```python
from build123d import *

# Parameters (mm, degrees)
SKETCH1_W                      = 912
SKETCH1_H                      = 225
BASE_FLANGE1_DEPTH             = 1.5
EDGE_FLANGE1_STRIP_W           = 10
EDGE_FLANGE1_STRIP_H           = 1.5
EDGE_FLANGE1_STRIP_CUT_DEPTH   = 912
EDGE_FLANGE1_STRIP_2_W         = 10
EDGE_FLANGE1_STRIP_2_H         = 1.5
EDGE_FLANGE1_STRIP_CUT_2_DEPTH = 912
EDGE_FLANGE1_DEPTH             = 912
EDGE_FLANGE1_BEND_DEPTH        = 912
EDGE_FLANGE2_STRIP_W           = 10
EDGE_FLANGE2_STRIP_H           = 1.5
EDGE_FLANGE2_STRIP_CUT_DEPTH   = 912
EDGE_FLANGE2_STRIP_2_W         = 10
EDGE_FLANGE2_STRIP_2_H         = 1.5
EDGE_FLANGE2_STRIP_CUT_2_DEPTH = 912
EDGE_FLANGE2_DEPTH             = 912
EDGE_FLANGE2_BEND_DEPTH        = 912
SKETCH18_R                     = 6
CUT_EXTRUDE1_DEPTH             = 280
SKETCH19_R                     = 6
CUT_EXTRUDE2_DEPTH             = 5


# Sheet-metal steps are written as plain solids
with BuildPart() as part:
    # Sketch1 → Base-Flange1 (new body)
    with BuildSketch(Plane(origin=(0, 0, 0), x_dir=(1, 0, 0), z_dir=(0, 1, 0))):
        Rectangle(SKETCH1_W, SKETCH1_H)
    extrude(amount=-BASE_FLANGE1_DEPTH)

    # Edge-Flange1 strip (across the edge) → Edge-Flange1 strip cut (cut)
    with BuildSketch(Plane(origin=(-456, 0, 112.5), x_dir=(0, 0, -1), z_dir=(1, 0, 0))):
        with Locations((-1.5, -0.75)):
            Rectangle(EDGE_FLANGE1_STRIP_W, EDGE_FLANGE1_STRIP_H)
    extrude(amount=EDGE_FLANGE1_STRIP_CUT_DEPTH, mode=Mode.SUBTRACT)

    # Edge-Flange1 strip 2 (across the edge) → Edge-Flange1 strip cut 2 (cut)
    with BuildSketch(Plane(origin=(456, 0, -112.5), x_dir=(0, 0, 1), z_dir=(-1, 0, 0))):
        with Locations((-1.5, -0.75)):
            Rectangle(EDGE_FLANGE1_STRIP_2_W, EDGE_FLANGE1_STRIP_2_H)
    extrude(amount=EDGE_FLANGE1_STRIP_CUT_2_DEPTH, mode=Mode.SUBTRACT)

    # Edge-Flange1 section (across the edge) → Edge-Flange1 (add)
    with BuildSketch(Plane(origin=(-456, 0, 112.5), x_dir=(0, 0, -1), z_dir=(1, 0, 0))):
        with BuildLine():
            Line((0, 2), (0, 38.5))
            Line((0, 38.5), (1.5, 38.5))
            Line((1.5, 38.5), (1.5, 2))
            ThreePointArc((1.5, 2), (2.085786438, 0.585786438), (3.5, 0))
            Line((3.5, 0), (3.5, -1.5))
            ThreePointArc((3.5, -1.5), (1.025126266, -0.474873734), (0, 2))
        make_face()
    extrude(amount=EDGE_FLANGE1_DEPTH)

    # Edge-Flange1 section 2 (across the edge) → Edge-Flange1 bend (add)
    with BuildSketch(Plane(origin=(456, 0, -112.5), x_dir=(0, 0, 1), z_dir=(-1, 0, 0))):
        with BuildLine():
            Line((0, 2), (0, 38.5))
            Line((0, 38.5), (1.5, 38.5))
            Line((1.5, 38.5), (1.5, 2))
            ThreePointArc((1.5, 2), (2.085786438, 0.585786438), (3.5, 0))
            Line((3.5, 0), (3.5, -1.5))
            ThreePointArc((3.5, -1.5), (1.025126266, -0.474873734), (0, 2))
        make_face()
    extrude(amount=EDGE_FLANGE1_BEND_DEPTH)

    # Edge-Flange2 strip (across the edge) → Edge-Flange2 strip cut (cut)
    with BuildSketch(Plane(origin=(-456, 38.5, 111), x_dir=(0, -1, 0), z_dir=(1, 0, 0))):
        with Locations((-1.5, -0.75)):
            Rectangle(EDGE_FLANGE2_STRIP_W, EDGE_FLANGE2_STRIP_H)
    extrude(amount=EDGE_FLANGE2_STRIP_CUT_DEPTH, mode=Mode.SUBTRACT)

    # Edge-Flange2 strip 2 (across the edge) → Edge-Flange2 strip cut 2 (cut)
    with BuildSketch(Plane(origin=(456, 38.5, -111), x_dir=(0, -1, 0), z_dir=(-1, 0, 0))):
        with Locations((-1.5, -0.75)):
            Rectangle(EDGE_FLANGE2_STRIP_2_W, EDGE_FLANGE2_STRIP_2_H)
    extrude(amount=EDGE_FLANGE2_STRIP_CUT_2_DEPTH, mode=Mode.SUBTRACT)

    # Edge-Flange2 section (across the edge) → Edge-Flange2 (add)
    with BuildSketch(Plane(origin=(-456, 38.5, 111), x_dir=(0, -1, 0), z_dir=(1, 0, 0))):
        with BuildLine():
            Line((0, 2), (0, 36.5))
            Line((0, 36.5), (1.5, 36.5))
            Line((1.5, 36.5), (1.5, 2))
            ThreePointArc((1.5, 2), (2.085786438, 0.585786438), (3.5, 0))
            Line((3.5, 0), (3.5, -1.5))
            ThreePointArc((3.5, -1.5), (1.025126266, -0.474873734), (0, 2))
        make_face()
    extrude(amount=EDGE_FLANGE2_DEPTH)

    # Edge-Flange2 section 2 (across the edge) → Edge-Flange2 bend (add)
    with BuildSketch(Plane(origin=(456, 38.5, -111), x_dir=(0, -1, 0), z_dir=(-1, 0, 0))):
        with BuildLine():
            Line((0, 2), (0, 36.5))
            Line((0, 36.5), (1.5, 36.5))
            Line((1.5, 36.5), (1.5, 2))
            ThreePointArc((1.5, 2), (2.085786438, 0.585786438), (3.5, 0))
            Line((3.5, 0), (3.5, -1.5))
            ThreePointArc((3.5, -1.5), (1.025126266, -0.474873734), (0, 2))
        make_face()
    extrude(amount=EDGE_FLANGE2_BEND_DEPTH)

    # Sketch18 → Cut-Extrude1 (cut)
    with BuildSketch(Plane.XY.offset(112.5)):
        with Locations((380, 18.5)):
            Circle(SKETCH18_R)
        with Locations((228, 18.5)):
            Circle(SKETCH18_R)
        with Locations((76, 18.5)):
            Circle(SKETCH18_R)
        with Locations((-76, 18.5)):
            Circle(SKETCH18_R)
        with Locations((-228, 18.5)):
            Circle(SKETCH18_R)
        with Locations((-380, 18.5)):
            Circle(SKETCH18_R)
    extrude(amount=-CUT_EXTRUDE1_DEPTH, mode=Mode.SUBTRACT)

    # Sketch19 → Cut-Extrude2 (cut)
    with BuildSketch(Plane(origin=(0, 38.5, 0), x_dir=(1, 0, 0), z_dir=(0, 1, 0))):
        with Locations(Location((-380, -91.75, 0), (0, 0, 270))):
            Circle(SKETCH19_R)
        with Locations(Location((-228, -91.75, 0), (0, 0, 270))):
            Circle(SKETCH19_R)
        with Locations(Location((-76, -91.75, 0), (0, 0, 270))):
            Circle(SKETCH19_R)
        with Locations(Location((76, -91.75, 0), (0, 0, 270))):
            Circle(SKETCH19_R)
        with Locations(Location((228, -91.75, 0), (0, 0, 270))):
            Circle(SKETCH19_R)
        with Locations(Location((380, -91.75, 0), (0, 0, 270))):
            Circle(SKETCH19_R)
        with Locations(Location((380, 91.75, 0), (0, 0, 90))):
            Circle(SKETCH19_R)
        with Locations(Location((228, 91.75, 0), (0, 0, 90))):
            Circle(SKETCH19_R)
        with Locations(Location((76, 91.75, 0), (0, 0, 90))):
            Circle(SKETCH19_R)
        with Locations(Location((-76, 91.75, 0), (0, 0, 90))):
            Circle(SKETCH19_R)
        with Locations(Location((-228, 91.75, 0), (0, 0, 90))):
            Circle(SKETCH19_R)
        with Locations(Location((-380, 91.75, 0), (0, 0, 90))):
            Circle(SKETCH19_R)
    extrude(amount=-CUT_EXTRUDE2_DEPTH, mode=Mode.SUBTRACT)


solid = part.part
```
Can you work these out from the model? Positions are in its coordinate system, mm. A direction names the side the tool comes from. Give positions to 0.01 mm unless a question says otherwise; leave off trailing zeros. Order: outer loops, then holes, each group sorted by start corner. A loop starts at its lowest first (then second) coordinate and runs counter-clockwise, first axis right, second up. Notation, with made-up numbers: (46, 79.25) - (80, 79.25) arc R5 cw to (80, 84.25) - close; hole circle Ø4 at (86, 55.5). An arc over 180 degrees is marked (long way). Use a Markdown table: item, result. Add a question column.
Q1. If we section it at A-A on x = -98: Write out the boundary of the cut face in (y, z), plus the area to 3 significant figures.
Q2. Please list where these lines run through material, in increasing order: line 1 along Y through (x, z) = (-382, 79); line 2 along Z through (x, y) = (-334.5, 20); line 3 along Z through (x, y) = (279, 36).
Q3. On a 3-axis mill with a long thin cutter (end or side, diameter ignored), from which of +Z, -Z, +X, -X, +Y, -Y can I reach the whole of each face in a straight line? I mean faces 4 (the flat face through (-6, 19, 111)), 5 (the flat face through (-6, 18, 112.5)). Say none if no direction works.
Q4. If we section it at C-C on z = -52.5: Write out the boundary of the cut face in (x, y), plus the area to 3 significant figures.
Q5. If we mould it in two halves opening along Y, with no side actions, what happens to faces 1 (the flat face through (-6, -1.5, -2)), 2 (the flat face through (-456, -1, 1)), 3 (the flat face through (-6, 0, -2))? For each: released by +Y, released by -Y, zero draft, split by the parting line, or undercut.
Q6. I'm going to push flat-ended pins straight in: pin 1 (0.8 mm diameter, centred on x = 22, y = 37.5, fed in from -Z); pin 2 (7 mm diameter, centred on x = 380, y = 18.5, fed in from +Z); pin 3 (4 mm diameter, centred on x = -89.5, z = -1.5, fed in from +Y). Where does each tip first touch, or does it pass through?
Q7. If we section it at B-B on y = 18.5: Count the separate pieces of the cut face and the enclosed holes in it, plus the area to 3 significant figures.
Answers follow:
| question | item | result |
|---|---|---|
| 1 | outline | (-1.5, -109) arc R3.5 ccw to (2, -112.5) - (35, -112.5) arc R3.5 ccw to (38.5, -109) - (38.5, -74.5) - (37, -74.5) - (37, -109) arc R2 cw to (35, -111) - (2, -111) arc R2 cw to (0, -109) - (0, 109) arc R2 cw to (2, 111) - (35, 111) arc R2 cw to (37, 109) - (37, 74.5) - (38.5, 74.5) - (38.5, 109) arc R3.5 ccw to (35, 112.5) - (2, 112.5) arc R3.5 ccw to (-1.5, 109) - close |
| 1 | area | 555 mm^2 |
| 2 | line 1 | y = -1.5 to 0, 37 to 38.5 |
| 2 | line 2 | z = -112.5 to -111, 111 to 112.5 |
| 2 | line 3 | z = -112.35 to -110.73, 110.73 to 112.35 |
| 3 | face 4 | +X, -X |
| 3 | face 5 | +Z, +X, -X, +Y, -Y |
| 4 | outline | (-456, -1.5) - (456, -1.5) - (456, 0) - (-456, 0) - close |
| 4 | area | 1,370 mm^2 |
| 5 | face 1 | released by -Y |
| 5 | face 2 | zero draft |
| 5 | face 3 | undercut |
| 6 | pin 1 | stops at z = -111.8 |
| 6 | pin 2 | passes through |
| 6 | pin 3 | stops at y = 0 |
| 7 | separate pieces | 14 |
| 7 | enclosed holes | 0 |
| 7 | area | 2,520 mm^2 |
